Study the drawing (mm; zero at the part's minimum x, y, z) and answer. Coordinates: 2 decimals unless noted, no trailing zeros. Loops run counter-clockwise (first coordinate to the right, second up) from the corner with the lowest first, then second, coordinate; pieces in that order, holes last. Notation, with made-up numbers: (37, 69.25) - (72, 69.25) arc R26 cw to (72, 98.25) - close; hole circle Ø9 at (28, -28). An arc over 180 degrees is marked (long way). Write each question's results on one line, items separated by ' | '. Start each with the question number.
(1) Determine the mould class of the marked faces 1, 2 and 3 for opening direction X: released by +X, released by -X, zero draft, split by the parting line, or undercut.
(2) Consider line 1 (X direction, y = 10, z = 50); line 2 (X direction, y = 15.5, z = 20.5); line 3 (Z direction, x = 5, y = 1.5). Determine where each line is inside the solid, lowest interval first. Write a range as from..to.
(3) Given pin 1 Ø10 at (x, z) = (11, 34) entering from +Y; pin 2 Ø8 at (x, y) = (9, 13) entering from -Z; pin 3 Ø2 at (x, z) = (3.5, 50.5) entering from -Y (1 decimal), each flat-ended and moving along its own axis, determine where each tip first touches the part or whether it passes through.
(4) Find section B-B on x = 12.5. Determine the outline of the cut face in (y, z).
(5) Find section C-C on y = 15.75. Determine the outline of the cut face in (x, z).
(6) Find section D-D on y = 1.5. Determine the outline of the cut face in (x, z).
(7) Find section A-A on z = 40.5. Determine the outline of the cut face in (x, y).
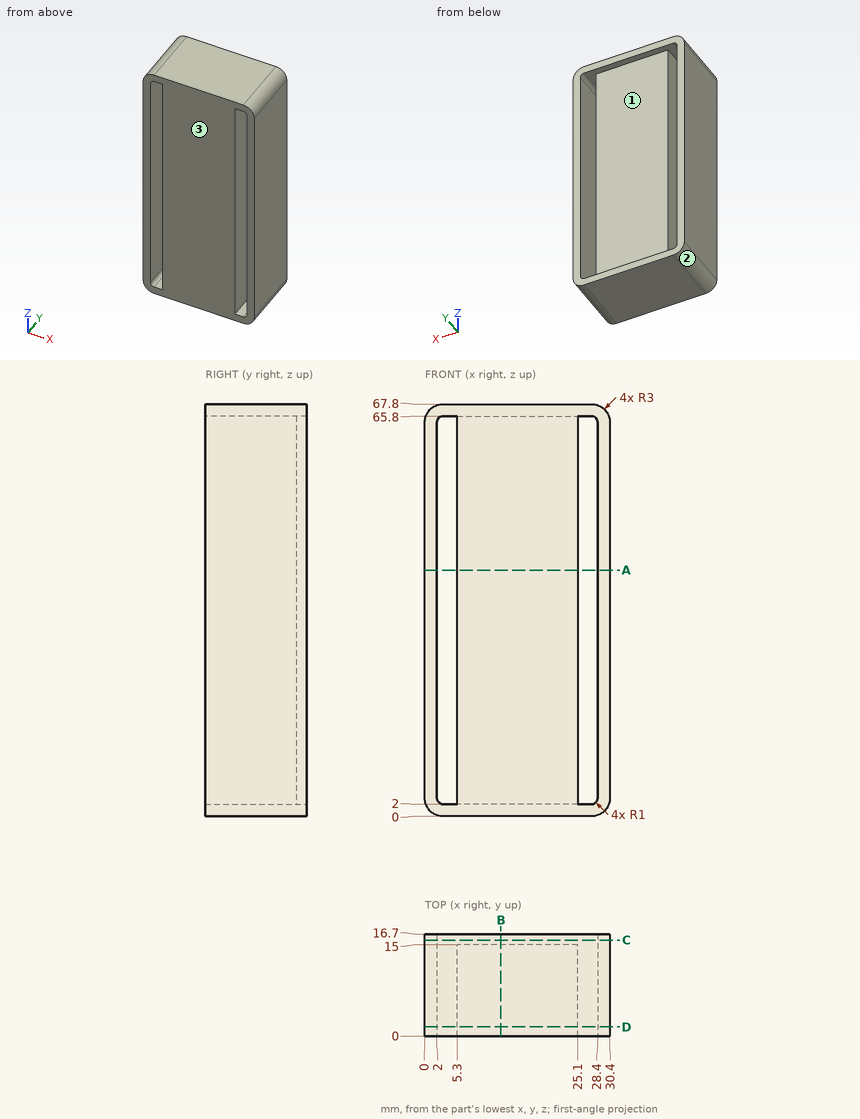
Values:
1) face 1: undercut | face 2: released by -X | face 3: zero draft
2) line 1: x = 0..2, 5.3..25.1, 28.4..30.4 | line 2: x = 0..2, 28.4..30.4 | line 3: z = 0..2, 65.8..67.8
3) pin 1: stops at y = 15 | pin 2: stops at z = 0 | pin 3: passes through
4) outline: (0, 0) - (16.7, 0) - (16.7, 2) - (15, 2) - (15, 65.8) - (16.7, 65.8) - (16.7, 67.8) - (0, 67.8) - close
5) outline: (0, 3) arc R3 ccw to (3, 0) - (27.4, 0) arc R3 ccw to (30.4, 3) - (30.4, 64.8) arc R3 ccw to (27.4, 67.8) - (3, 67.8) arc R3 ccw to (0, 64.8) - close; hole (2, 3) arc R1 ccw to (3, 2) - (27.4, 2) arc R1 ccw to (28.4, 3) - (28.4, 64.8) arc R1 ccw to (27.4, 65.8) - (3, 65.8) arc R1 ccw to (2, 64.8) - close
6) outline: (0, 3) arc R3 ccw to (3, 0) - (27.4, 0) arc R3 ccw to (30.4, 3) - (30.4, 64.8) arc R3 ccw to (27.4, 67.8) - (3, 67.8) arc R3 ccw to (0, 64.8) - close; hole (2, 3) arc R1 ccw to (3, 2) - (5.3, 2) - (5.3, 65.8) - (3, 65.8) arc R1 ccw to (2, 64.8) - close; hole (25.1, 2) - (27.4, 2) arc R1 ccw to (28.4, 3) - (28.4, 64.8) arc R1 ccw to (27.4, 65.8) - (25.1, 65.8) - close
7) outline: (0, 0) - (2, 0) - (2, 16.7) - (0, 16.7) - close; (5.3, 0) - (25.1, 0) - (25.1, 15) - (5.3, 15) - close; (28.4, 0) - (30.4, 0) - (30.4, 16.7) - (28.4, 16.7) - close
